Verification items for the finished model (mm, model axes). A direction names the side the tool comes from. Give positions to 0.01 mm unless a question says otherwise; leave off trailing zeros. Write each loop counter-clockwise with the first axis right and the second up, starting at its lowest first coordinate (ties: lowest second). Pieces come first, ordered by that corner, then holes. Notation, with made-up numbers: M -15.5,12 L 32.5,12 A29 cw 32.5,33 Z; hole C 20.25,33.25 d1. An arc over 180 degrees is marked long. Answer as a JSON object with one key per item and string values.
```python
from build123d import *

# Parameters (mm, degrees)
SKETCH3_R           = 34
SKETCH3_R_2         = 10.9
BOSS_EXTRUDE2_DEPTH = 1
SKETCH4_R           = 34
SKETCH4_R_2         = 3.925
BOSS_EXTRUDE3_DEPTH = 4


with BuildPart() as part:
    # Sketch3 → Boss-Extrude2 (new body)
    with BuildSketch(Plane.XY):
        with Locations((9.62, 10)):
            Circle(SKETCH3_R)
        with Locations((9.62, 10)):
            Circle(SKETCH3_R_2, mode=Mode.SUBTRACT)
    extrude(amount=-BOSS_EXTRUDE2_DEPTH)

    # Sketch4 → Boss-Extrude3 (add)
    with BuildSketch(Plane.XY):
        with Locations((9.62, 10)):
            Circle(SKETCH4_R)
        with Locations((9.62, 10)):
            Circle(SKETCH4_R_2, mode=Mode.SUBTRACT)
    extrude(amount=BOSS_EXTRUDE3_DEPTH)


solid = part.part
```
1) Access from +Z, -Z, +X, -X, +Y, -Y to the whole of each face (thin tool, end or side, straight path). Record for faces 1 (the face through (9, 5, 0)), 2 (the face through (8.77, 6.17, 1.97)).
Completed:
{"face 1": "-Z", "face 2": "+Z, -Z"}
2) Section check A-A on x = 9.62. Record the boundary of the cut face in (y, z) (3 decimals), and give its area (3 significant figures).
Completed:
{"outline": "M -24,-1 L -0.9,-1 L -0.9,0 L 6.075,0 L 6.075,4 L -24,4 Z; M 13.925,0 L 20.9,0 L 20.9,-1 L 44,-1 L 44,4 L 13.925,4 Z", "area": "287 mm2"}
3) Release check for a two-part mould opening along Y. For faces 3 (the face through (1.6, 18, -1)), 4 (the face through (7.26, -0.64, -0.49)) record: pulls with the +Y half, pulls with the -Y half, needs draft (parallel to the pull), parting line crosses it, or undercut.
Completed:
{"face 3": "needs draft", "face 4": "undercut"}
4) Thickness scan on L1, parallel to Y at x = 9.62, z = -0.45; L2, parallel to Y at x = 9.62, z = 2.2 (3 decimals); L3, parallel to X at y = 12, z = 1.1. Record the ranges inside material, lowest first.
Completed:
{"L1": "y = -24 to -0.9, 20.9 to 44", "L2": "y = -24 to 6.075, 13.925 to 44", "L3": "x = -24.32 to 6.24, 13 to 43.56"}
5) Section check D-D on y = 19. Record the boundary of the cut face in (x, z).
Completed:
{"outline": "M -23.17,-1 L 3.47,-1 L 3.47,0 L 15.77,0 L 15.77,-1 L 42.41,-1 L 42.41,4 L -23.17,4 Z"}
6) Section check B-B on y = 10. Record the boundary of the cut face in (x, z) (3 decimals), and give its area (3 significant figures).
Completed:
{"outline": "M -24.38,-1 L -1.28,-1 L -1.28,0 L 5.695,0 L 5.695,4 L -24.38,4 Z; M 13.545,0 L 20.52,0 L 20.52,-1 L 43.62,-1 L 43.62,4 L 13.545,4 Z", "area": "287 mm2"}
7) Section check C-C on z = 1.8. Record the boundary of the cut face in (x, y) (3 decimals).
Completed:
{"outline": "C 9.62,10 d68; hole C 9.62,10 d7.85"}
8) Go/stop test with flat-tipped pins: pin 1 (2 mm diameter, centred on y = -15, z = 3.5, fed in from +X); pin 2 (6.5 mm diameter, centred on x = 8.5, y = 13.5, fed in from -Z); pin 3 (1.5 mm diameter, centred on y = -2.5, z = 3, fed in from +X); pin 4 (6.5 mm diameter, centred on x = 9.62, y = 10, fed in from +Z). Record where each tip stops, or that it passes through.
Completed:
{"pin 1": "stops at x = 33.7", "pin 2": "stops at z = 0", "pin 3": "stops at x = 41.53", "pin 4": "passes through"}
